```python
from build123d import *

# Parameters (mm, degrees)
ESBO_O1_W                = 50
ESBO_O1_H                = 100
RESSALTO_EXTRUS_O1_DEPTH = 3.125
ESBO_O2_R                = 16
CORTE_EXTRUS_O1_DEPTH    = 3.125


with BuildPart() as part:
    # Esboço1 → Ressalto-extrusão1 (new body)
    with BuildSketch(Plane.XY):
        with Locations((-25, 50)):
            Rectangle(ESBO_O1_W, ESBO_O1_H)
    extrude(amount=RESSALTO_EXTRUS_O1_DEPTH)

    # Esboço2 → Corte-extrusão1 (cut)
    with BuildSketch(Plane.XY.offset(3.125)):
        with Locations((-25, 79.712786513)):
            Circle(ESBO_O2_R)
        with BuildLine():
            Line((-36.464726097, 35), (-36.464726097, 0))
            Line((-36.464726097, 0), (-40.464726097, 0))
            Line((-40.464726097, 0), (-40.464726097, 35))
            ThreePointArc((-40.464726097, 35), (-38.464726097, 37), (-36.464726097, 35))
        make_face()
        with BuildLine():
            Line((-13.535273903, 35), (-13.535273903, 0))
            Line((-13.535273903, 0), (-9.535273903, 0))
            Line((-9.535273903, 0), (-9.535273903, 35))
            ThreePointArc((-9.535273903, 35), (-11.535273903, 37), (-13.535273903, 35))
        make_face()
    extrude(amount=-CORTE_EXTRUS_O1_DEPTH, mode=Mode.SUBTRACT)


solid = part.part
```
The model under review builds one solid part; all positions refer to its coordinate system, in mm. A direction names the side the tool comes from. Round coordinates to 2 decimals unless told otherwise and drop trailing zeros. Loops run counter-clockwise (first coordinate to the right, second up) from the corner with the lowest first, then second, coordinate; pieces in that order, holes last. Notation, with made-up numbers: (28, 14) - (83, 14) arc R15 ccw to (83, 32) - close; hole circle Ø6 at (89, -15.75). An arc over 180 degrees is marked (long way). Write each question's results on one line, items separated by ' | '. Start each with the question number.
Q1. Wall thickness on line 1 along X through (y, z) = (16, 1.7); line 2 along Y through (x, z) = (-25, 1.8); line 3 along Y through (x, z) = (-37, 2.4): over which ranges is each line inside the solid? List them lowest first. Write a range as [from, to].
Q2. Take a section at A-A on x = -25. Give the boundary of the cut face in (y, z) (3 decimals), plus the area to 4 significant figures.
Q3. Take a section at C-C on z = 0.7. Give the boundary of the cut face in (x, y), plus the area to 3 significant figures.
Q4. Tool access review of faces 1 (the flat face through (-40.465, 17, 2)), 2 (the flat face through (-45, 0, 2)): name each direction out of +Z, -Z, +X, -X, +Y, -Y from which nothing blocks a thin tool from reaching the whole face with its end or side.
Q5. Take a section at B-B on y = 67. Give the boundary of the cut face in (x, z) (3 decimals), plus the area to 3 significant figures.
Q6. Draft analysis for pull direction X (two halves, no side actions). For faces 3 (the flat face through (-5, 0, 2)), 4 (the flat face through (-36.465, 18, 2)), 5 (the flat face through (-50, 49, 2)), state which applies: pulls with the +X half, pulls with the -X half, needs draft (parallel to the pull), parting line crosses it, or undercut.
Data:
1) line 1: x = [-50, -40.46], [-36.46, -13.54], [-9.54, 0] | line 2: y = [0, 63.71], [95.71, 100] | line 3: y = [36.36, 69.13], [90.3, 100]
2) outline: (0, 0) - (63.713, 0) - (63.713, 3.125) - (0, 3.125) - close; (95.713, 0) - (100, 0) - (100, 3.125) - (95.713, 3.125) - close | area: 212.5 mm²
3) outline: (-50, 0) - (-40.46, 0) - (-40.46, 35) arc R2 cw to (-36.46, 35) - (-36.46, 0) - (-13.54, 0) - (-13.54, 35) arc R2 cw to (-9.54, 35) - (-9.54, 0) - (0, 0) - (0, 100) - (-50, 100) - close; hole circle Ø32 at (-25, 79.71) | area: 3,900 mm²
4) face 1: +Z, -Z, -Y | face 2: +Z, -Z, +X, -X, -Y
5) outline: (-50, 0) - (-34.715, 0) - (-34.715, 3.125) - (-50, 3.125) - close; (-15.285, 0) - (0, 0) - (0, 3.125) - (-15.285, 3.125) - close | area: 95.5 mm²
6) face 3: needs draft | face 4: undercut | face 5: pulls with the -X half
